The listing builds one solid part. Answer for the finished solid, in the listing's coordinates (mm). Round coordinates to 2 decimals unless told otherwise and drop trailing zeros. Write each loop counter-clockwise with the first axis right and the second up, starting at its lowest first coordinate (ties: lowest second). Pieces come first, ordered by that corner, then holes. Notation, with made-up numbers: (84, -25) - (141, -25) arc R16 cw to (141, -5) - close; hole circle Ø5 at (-32, 67.5). An arc over 180 degrees is marked (long way). Return JSON: item names as keys, results as strings. Group by question number.
(1) Section B-B, the plane y = 212.5 is taken. Write down the section's boundary in (x, z).
(2) Section A-A, the plane x = 1.9 is taken. Write down the section's boundary in (y, z), then the cut area to 3 significant figures.
(3) Find the intervals of material crossed by line 1 along Y through (x, z) = (0.45, 353.5); line 2 along Y through (x, z) = (3.1, 118.5), in increasing order. Write a range as [from, to].
(4) Each of these flat-tipped pins is pushed along its axis until it touches: pin 1 (2 mm diameter, centred on x = 3, z = 3.5, fed in from +Y); pin 2 (2 mm diameter, centred on x = 3, z = 280.5, fed in from +Y); pin 3 (1.3 mm diameter, centred on x = 3, z = 354, fed in from +Y). Where does it stop, or does it pass through?
```python
from build123d import *

# Parameters (mm, degrees)
SKETCH2_R           = 2
BOSS_EXTRUDE1_DEPTH = 4.5
SKETCH3_R           = 2
CUT_EXTRUDE1_DEPTH  = 459.798975587
FILLET2_R           = 0.5
FILLET4_R           = 0.5
FILLET5_R           = 0.5
FILLET6_R           = 3
FILLET7_R           = 3
FILLET8_R           = 1


with BuildPart() as part:
    # Sketch2 → Boss-Extrude1 (new body)
    with BuildSketch(Plane(origin=(0, 0, 0), x_dir=(0, 0, -1), z_dir=(1, 0, 0))):
        Polygon((-30, 30), (-30, 248.5), (-24, 248.5), (-24, 268.5), (-12, 268.5), (-12, 248.5), (0, 248.5), (0, 0), (-372, 0), (-372, 30), (-360, 30), (-360, 10), (-348, 10), (-348, 30), align=None)
        with Locations((-12, 12)):
            Circle(SKETCH2_R, mode=Mode.SUBTRACT)
    extrude(amount=BOSS_EXTRUDE1_DEPTH)

    # Sketch3 → Cut-Extrude1 (cut, through all)
    with BuildSketch(Plane(origin=(4.5, 0, 0), x_dir=(0, 0, -1), z_dir=(1, 0, 0))):
        with Locations((-12, 266.5)):
            Circle(SKETCH3_R)
        with Locations((-360, 12)):
            Circle(SKETCH3_R)
    extrude(amount=-CUT_EXTRUDE1_DEPTH, mode=Mode.SUBTRACT)

    # Fillet2
    fillet2_edges = [part.edges().sort_by_distance(p)[0] for p in [
        (2.25, 264.5, 12),
    ]]
    fillet(fillet2_edges, radius=FILLET2_R)

    # Fillet4
    fillet4_edges = [part.edges().sort_by_distance(p)[0] for p in [
        (2.25, 268.5, 12),
    ]]
    fillet(fillet4_edges, radius=FILLET4_R)

    # Fillet5
    fillet5_edges = [part.edges().sort_by_distance(p)[0] for p in [
        (2.25, 14, 360),
    ]]
    fillet(fillet5_edges, radius=FILLET5_R)

    # Fillet6
    fillet6_edges = [part.edges().sort_by_distance(p)[0] for p in [
        (2.25, 30, 360),
        (2.25, 30, 348),
        (2.25, 248.5, 24),
        (2.25, 248.5, 12),
    ]]
    fillet(fillet6_edges, radius=FILLET6_R)

    # Fillet7
    fillet7_edges = [part.edges().sort_by_distance(p)[0] for p in [
        (2.25, 10, 348),
        (2.25, 268.5, 24),
    ]]
    fillet(fillet7_edges, radius=FILLET7_R)

    # Fillet8
    fillet8_edges = [part.edges().sort_by_distance(p)[0] for p in [
        (2.25, 0, 0),
        (2.25, 0, 372),
    ]]
    fillet(fillet8_edges, radius=FILLET8_R)


solid = part.part
```
Working result:
{
 "1": {"outline": "(0, 0) - (4.5, 0) - (4.5, 30) - (0, 30) - close"},
 "2": {"outline": "(0, 1) arc R1 ccw to (1, 0) - (248.5, 0) - (248.5, 9) arc R3 cw to (251.5, 12) - (264.05, 12) arc R0.5 ccw to (264.54, 12.4) arc R2 cw to (267.7, 13.6) arc R0.5 ccw to (268.5, 14) - (268.5, 21) arc R3 ccw to (265.5, 24) - (251.5, 24) arc R3 cw to (248.5, 27) - (248.5, 30) - (30, 30) - (30, 345) arc R3 ccw to (27, 348) - (13, 348) arc R3 cw to (10, 351) - (10, 360) arc R2 cw to (13.96, 360.4) arc R0.5 ccw to (14.45, 360) - (27, 360) arc R3 ccw to (30, 363) - (30, 372) - (1, 372) arc R1 ccw to (0, 371) - close; hole circle Ø4 at (12, 12)", "area": "17,700 mm^2"},
 "3": {"line 1": "y = [0, 10]", "line 2": "y = [0, 30]"},
 "4": {"pin 1": "stops at y = 248.5", "pin 2": "stops at y = 30", "pin 3": "stops at y = 10"}
}
